Geometry: final body of the model. Coordinates: model frame, mm. A direction names the side the tool comes from. Round coordinates to 2 decimals unless told otherwise and drop trailing zeros. Order: outer loops, then holes, each group sorted by start corner. A loop starts at its lowest first (then second) coordinate and runs counter-clockwise, first axis right, second up. Notation, with made-up numbers: M 65,9.25 L 94,9.25 A21 ccw 94,18.25 Z; hole C 5,9 d5. An arc over 180 degrees is marked long. Put each result on its own line as item: value. Start each with the question number.
1) Section B-B, the plane z = -226.5. Return loops of the section in (x, y), then the cut area to 3 significant figures.
2) First-contact query: P1, Ø3.5, axis at x = 0, y = 0, coming from the -Z side. Flat tip, straight axial feed; report the tip coordinate or a pass-through.
3) Access query for faces 1 (the cylindrical face through (-33, 0, -138)), 2 (the flat face through (1, -2, 0)). Directions: +Z, -Z, +X, -X, +Y, -Y. A direction counts if a zero-diameter tool reaches every point of the face in a straight line with its end or side. Return the directions, or none.
4) Draft query along Z for faces 3 (the cylindrical face through (-3, 0, -142)), 4 (the flat face through (-38, -1, 0)). Return one class per face: pulls with the +Z half, pulls with the -Z half, needs draft (parallel to the pull), parting line crosses it, or undercut.
5) Material intervals for probe 1 along X at (y, z) = (0, -167.5); probe 2 along X at (y, z) = (-0.75, -135); probe 3 along Y at (x, z) = (-36, -63), sorted ascending. Write a range as [from, to].
6) Section A-A, the plane y = 0. Return loops of the section in (x, z), then the cut area to 3 significant figures.
Autodesk Inventor part; units mm, degrees
ref_plane "YZ Plane" through (0, 0, 0) normal (1, 0, 0) x (0, 1, 0)
ref_plane "XZ Plane" through (0, 0, 0) normal (0, 1, 0) x (-1, 0, 0)
ref_plane "XY Plane" through (0, 0, 0) normal (0, 0, 1) x (1, 0, 0)
sketch "Sketch1" plane through (0, 0, 0) normal (0, 0, 1) x (1, 0, 0)
  line L0 (0, 4.2) -> (0, -4.2) construction
  line L1 (-4.2, 0) -> (4.2, 0) construction
  circle A0 centre (0, 0) radius 3
  circle A1 centre (0, 0) radius 2
  dimension "d4" = 6
  dimension "d5" = 4
sketch "Sketch2" plane through (0, 0, 0) normal (0, 1, 0) x (-1, 0, 0)
  line L0 (0, 0) -> (0, -280)
  arc A0 (0, -280) -> (36, -280) centre (18, -280) ccw
  line L1 (36, -280) -> (36, 0)
  dimension "d6" = 36
  dimension "d7" = 280
  dimension "d13" = 280
sweep "Sweep1" add profiles "Sketch1" path "Sketch2"
equation "\"d7\" = d13"
properties part number "17-0028-0022" material "Copper"
Result sheet:
1. outline: C -36,0 d6; C 0,0 d6; hole C -36,0 d4; hole C 0,0 d4
1. area: 31.4 mm2
2. P1: stops at z = -293.3
3. face 1: +Z
3. face 2: +Z, +X, -X, +Y, -Y
4. face 3: needs draft
4. face 4: pulls with the +Z half
5. probe 1: x = [-39, -38], [-34, -33], [-3, -2], [2, 3]
5. probe 2: x = [-38.9, -37.85], [-34.15, -33.1], [-2.9, -1.85], [1.85, 2.9]
5. probe 3: y = [-3, -2], [2, 3]
6. outline: M -39,-280 A21 ccw 3,-280 L 3,0 L 2,0 L 2,-280 A20 cw -38,-280 L -38,0 L -39,0 Z; M -34,-280 A16 ccw -2,-280 L -2,0 L -3,0 L -3,-280 A15 cw -33,-280 L -33,0 L -34,0 Z
6. area: 1,230 mm2
